For this review, take the finished solid that the model builds, in its own axes (mm). A direction names the side the tool comes from. Round coordinates to 2 decimals unless told otherwise and drop trailing zeros. Order: outer loops, then holes, each group sorted by start corner. A loop starts at its lowest first (then second) coordinate and runs counter-clockwise, first axis right, second up.
```python
from build123d import *

# Parameters (mm, degrees)
SKETCH2_W           = 53
SKETCH2_H           = 17.5
BOSS_EXTRUDE1_DEPTH = 29
BOSS_EXTRUDE2_DEPTH = 2.5
BOSS_EXTRUDE3_DEPTH = 2.4


with BuildPart() as part:
    # Sketch2 → Boss-Extrude1 (new body)
    with BuildSketch(Plane(origin=(0, 0, 0), x_dir=(1, 0, 0), z_dir=(0, 1, 0))):
        Rectangle(SKETCH2_W, SKETCH2_H)
        with BuildLine():
            add(Edge.make_bspline(
                [(-26.5, -8.75), (-31.844612433, -9.598662384), (-38.964801167, -6.953731951), (-38.5, 0)],
                knots=[0, 0, 0, 0, 1, 1, 1, 1], degree=3))
            add(Edge.make_bspline(
                [(-26.5, 8.75), (-31.844612433, 9.598662384), (-38.964801167, 6.953731951), (-38.5, 0)],
                knots=[0, 0, 0, 0, 1, 1, 1, 1], degree=3))
            Line((-26.5, 8.75), (-26.5, -8.75))
        make_face()
    extrude(amount=BOSS_EXTRUDE1_DEPTH)

    # Sketch3 → Boss-Extrude2 (add)
    with BuildSketch(Plane(origin=(0, 29, 0), x_dir=(1, 0, 0), z_dir=(0, 1, 0))):
        Polygon((-38.5, 6), (-36.365233695, 6), (-36.365233695, 0), (-38.5, 0), (-41.5, 0), (-41.5, 6), align=None)
    extrude(amount=BOSS_EXTRUDE2_DEPTH)

    # Sketch4 → Boss-Extrude3 (add)
    with BuildSketch(Plane.XZ):
        Polygon((-38.5, 6), (-36.365233695, 6), (-36.365233695, 0), (-38.5, 0), (-42.5, 0), (-42.5, 6), align=None)
    extrude(amount=BOSS_EXTRUDE3_DEPTH)


solid = part.part
```
Q1. Wall thickness on line 1 (Y direction, x = 1, z = -7.5); line 2 (Z direction, x = -12.5, y = 17); line 3 (X direction, y = 11, z = -6): over which ranges is each line inside the solid? List them lowest first.
Q2. Clearance check with flat-ended pins moving along their axes: pin 1 (1.9 mm diameter, centred on x = -39.5, y = -1, fed in from -Z); pin 2 (1 mm diameter, centred on x = 13.5, y = 20.5, fed in from -Z); pin 3 (8 mm diameter, centred on x = 9, y = 9.5, fed in from +Z); pin 4 (3 mm diameter, centred on y = 30, z = -4, fed in from +X). State where each tip first meets the part, or that it passes through.
Q3. Take a section at A-A, the plane x = 22. State the section outline as (y, z) points, plus the area to 4 significant figures.
Q4. Tool access review of faces 1 (the face through (0, 14, -8.75)), 2 (the face through (-36.365, 30, -3)), 3 (the face through (-39, 29, -3)): name each direction out of +Z, -Z, +X, -X, +Y, -Y from which nothing blocks a thin tool from reaching the whole face with its end or side.
Working result:
1. line 1: y = 0 to 29
1. line 2: z = -8.75 to 8.75
1. line 3: x = -36.37 to 26.5
2. pin 1: stops at z = 0
2. pin 2: stops at z = -8.75
2. pin 3: stops at z = 8.75
2. pin 4: stops at x = 26.5
3. outline: (0, -8.75) - (29, -8.75) - (29, 8.75) - (0, 8.75) - close
3. area: 507.5 mm2
4. face 1: -Z, +X, +Y, -Y
4. face 2: +Z, -Z, +X, +Y
4. face 3: -Z, -X, -Y
